Design review of the part built by this model. Coordinates are the model's own, in mm. Round coordinates to 2 decimals unless told otherwise and drop trailing zeros. Order: outer loops, then holes, each group sorted by start corner. A loop starts at its lowest first (then second) coordinate and runs counter-clockwise, first axis right, second up. Notation, with made-up numbers: (23, 65) - (74, 65) arc R11 ccw to (74, 80) - close; hole circle Ø8 at (48, -30.75). An arc over 180 degrees is marked (long way). Use CSV: the item, a comma, the result in double quotes.
from build123d import *

# Parameters (mm, degrees)
SKETCH1_W           = 10
SKETCH1_H           = 15
BOSS_EXTRUDE1_DEPTH = 2.5
CUT_EXTRUDE1_REACH  = 15.693
SKETCH2_R           = 2.5


with BuildPart() as part:
    # Sketch1 → Boss-Extrude1 (new body)
    with BuildSketch(Plane(origin=(0, 0, 0), x_dir=(1, 0, 0), z_dir=(0, 1, 0))):
        with BuildLine():
            ThreePointArc((-5, 7.5), (0, 12.5), (5, 7.5))
            Line((5, 7.5), (-5, 7.5))
        make_face()
        Rectangle(SKETCH1_W, SKETCH1_H)
        with BuildLine():
            Line((-5, -7.5), (5, -7.5))
            ThreePointArc((5, -7.5), (0, -12.5), (-5, -7.5))
        make_face()
    extrude(amount=BOSS_EXTRUDE1_DEPTH)

    # Sketch2 → Cut-Extrude1 (cut, up to next)
    with BuildSketch(Plane(origin=(0, 2.5, 0), x_dir=(1, 0, 0), z_dir=(0, 1, 0)), mode=Mode.PRIVATE) as cut_extrude1_sk1:
        with Locations(Location((0, 7.5, 0), (0, 0, 270))):
            Circle(SKETCH2_R)
    cut_extrude1_tool1 = extrude(cut_extrude1_sk1.sketch, amount=-CUT_EXTRUDE1_REACH, mode=Mode.PRIVATE) & part.part
    # Sketch2 → Cut-Extrude1 (cut, up to next)
    with BuildSketch(Plane(origin=(0, 2.5, 0), x_dir=(1, 0, 0), z_dir=(0, 1, 0)), mode=Mode.PRIVATE) as cut_extrude1_sk2:
        with Locations(Location((0, 0, 0), (0, 0, 270))):
            Circle(SKETCH2_R)
    cut_extrude1_tool2 = extrude(cut_extrude1_sk2.sketch, amount=-CUT_EXTRUDE1_REACH, mode=Mode.PRIVATE) & part.part
    add(cut_extrude1_tool1.solids().sort_by_distance((0, 2.5, -7.5))[0], mode=Mode.SUBTRACT)
    add(cut_extrude1_tool2.solids().sort_by_distance((0, 2.5, 0))[0], mode=Mode.SUBTRACT)


solid = part.part
1) We need section A-A (x = 0). Give the boundary of the cut face in (y, z).
Data:
outline,"(0, -12.5) - (2.5, -12.5) - (2.5, -10) - (0, -10) - close; (0, -5) - (2.5, -5) - (2.5, -2.5) - (0, -2.5) - close; (0, 2.5) - (2.5, 2.5) - (2.5, 12.5) - (0, 12.5) - close"
2) To check wall thickness, follow L1, parallel to Z at x = -1.75, y = 1.4; L2, parallel to X at y = 1.5, z = 0; L3, parallel to Z at x = 1.25, y = 0.6. State the ranges of each line that lie inside material, in increasing order. Write a range as from..to.
Data:
L1,"z = -12.18..-9.29, -5.71..-1.79, 1.79..12.18"
L2,"x = -5..-2.5, 2.5..5"
L3,"z = -12.34..-9.67, -5.33..-2.17, 2.17..12.34"
3) We need section B-B (z = 0). Give the boundary of the cut face in (x, y).
Data:
outline,"(-5, 0) - (-2.5, 0) - (-2.5, 2.5) - (-5, 2.5) - close; (2.5, 0) - (5, 0) - (5, 2.5) - (2.5, 2.5) - close"
4) We need section C-C (y = 1.4). Give the boundary of the cut face in (x, z), then the cut area to 3 significant figures.
Data:
outline,"(-5, -7.5) arc R5 ccw to (5, -7.5) - (5, 7.5) arc R5 ccw to (-5, 7.5) - close; hole circle Ø5 at (0, -7.5); hole circle Ø5 at (0, 0)"
area,"189 mm2"
5) Insertion check: pin 1 Ø4 at (x, z) = (0, 0) entering from +Y; pin 2 Ø1.5 at (x, y) = (-2, 2) entering from -Z. Each pin has a flat end and moves straight along its axis. Give the tip position at first contact, or say it passes through.
Data:
pin 1,"passes through"
pin 2,"stops at z = -12.34"
6) We need section D-D (x = -2). Give the boundary of the cut face in (y, z).
Data:
outline,"(0, -12.08) - (2.5, -12.08) - (2.5, -9) - (0, -9) - close; (0, -6) - (2.5, -6) - (2.5, -1.5) - (0, -1.5) - close; (0, 1.5) - (2.5, 1.5) - (2.5, 12.08) - (0, 12.08) - close"
7) The part is to be moulded in two halves that separate along X. For faces 1 (the face through (0, 1, -10)), 2 (the face through (-2.44, 1.27, -0.54)), 3 (the face through (0, 0, 3)), 4 (the face through (-5, 1, 0)), say which applies: +X half, -X half, draft (parallel to the pull), parting line (faces both ways), or undercut.
Data:
face 1,"undercut"
face 2,"undercut"
face 3,"draft"
face 4,"-X half"
